from build123d import *

# Parameters (mm, degrees)
F1_DEPTH = 63.5
F2_DEPTH = 25.4
F3_DEPTH = 7.9375
F5_R     = 6.35


with BuildPart() as f1:
    # F0 (on Front) → F1 (new body, symmetric)
    with BuildSketch(Plane.XZ):
        Polygon((-41.275, -9.525), (41.275, -9.525), (41.275, 9.525), (22.225, 9.525), (-41.275, 9.525), align=None)
    extrude(amount=F1_DEPTH, both=True)

    # F0 (on Front) → F2 (join, symmetric)
    with BuildSketch(Plane.XZ):
        with BuildLine():
            Line((22.225, 9.525), (41.275, 9.525))
            Line((41.275, 9.525), (41.275, 27.0002))
            ThreePointArc((41.275, 27.0002), (45.9246798487, 38.2255201513), (57.15, 42.8752))
            Line((57.15, 42.8752), (60.325, 42.8752))
            Line((60.325, 42.8752), (60.325, 61.9252))
            Line((60.325, 61.9252), (57.15, 61.9252))
            add(Edge.make_bspline(
                [(53.8183914721, 61.765930391), (54.9540123477, 61.8314994044), (56.0654467047, 61.8844891287), (57.15, 61.9252)],
                knots=[108.0492715446, 108.0492715446, 108.0492715446, 108.0492715446, 111.5045361635, 111.5045361635, 111.5045361635, 111.5045361635], degree=3))
            ThreePointArc((53.8183914721, 61.765930391), (31.3032201925, 50.4884864122), (22.225, 27.0002))
            Line((22.225, 27.0002), (22.225, 9.525))
        make_face()
        Polygon((60.325, 61.9252), (60.325, 42.8752), (60.325, 38.1), (85.725, 38.1), (85.5438719422, 66.675), (60.325, 66.675), align=None)
    extrude(amount=F2_DEPTH, both=True)

    # F0 (on Front) → F3 (join, symmetric)
    with BuildSketch(Plane.XZ):
        with BuildLine():
            add(Edge.make_bspline(
                [(-41.275, 9.525), (-40.856674268, 45.3642172034), (18.3064924153, 59.7155276242), (53.8183914721, 61.765930391)],
                knots=[0, 0, 0, 0, 108.0492715446, 108.0492715446, 108.0492715446, 108.0492715446], degree=3))
            Line((-41.275, 9.525), (22.225, 9.525))
            Line((22.225, 9.525), (22.225, 27.0002))
            ThreePointArc((22.225, 27.0002), (31.3032201925, 50.4884864122), (53.8183914721, 61.765930391))
        make_face()
    extrude(amount=F3_DEPTH, both=True)

    # F0 (on Front) → F4 (revolve)
    with BuildSketch(Plane.XZ):
        Polygon((85.5438719422, 66.675), (85.725, 38.1), (111.125, 38.1), (111.125, 66.675), align=None)
    revolve(axis=Axis((85.6344359711, 0, 52.3875), (-0.0063385623, 0, 0.9999799111)))

    # F5
    f5_edges = [f1.edges().sort_by_distance(p)[0] for p in [
        (41.275, -63.5, 0),
        (-41.275, -63.5, 0),
        (-41.275, 63.5, 0),
        (41.275, 63.5, 0),
    ]]
    fillet(f5_edges, radius=F5_R)


solid = f1.part
Input: part model. Units: mm. Frame: model coordinates. A direction names the side the tool comes from. Coordinates: 2 decimals unless noted, no trailing zeros. Loops run counter-clockwise (first coordinate to the right, second up) from the corner with the lowest first, then second, coordinate; pieces in that order, holes last. Notation, with made-up numbers: (88, -9) -> (102, -9) arc R21 cw to (102, 27) -> close; hole circle Ø6 at (-8, -35). An arc over 180 degrees is marked (long way). Write item = value, one per line. Start each with the question number.
Item 1: Cut plane B-B, the plane y = -31. Return loops of the section in (x, z) (3 decimals).
Item 2: First-contact query: P1, Ø2.5, axis at x = 59, y = 5, coming from the +Z side; P2, Ø8, axis at x = 45.5, z = 44.5, coming from the +Y side; P3, Ø6, axis at x = 95, z = 54, coming from the -Y side. Flat tips, straight axial feed; report the tip coordinate or a pass-through.
Item 3: Cut plane A-A, the plane z = 0. Return loops of the section in (x, y) (3 decimals), plus the area to 3 significant figures.
Item 4: Reachability of faces 5 (the face through (45.8, -0.4, 38.1)), 6 (the face through (66, -19, 38.1)), 7 (the face through (22.225, -17, 18)), 8 (the face through (31.547, 16.547, 50.754)), 9 (the face through (87.2, 0.5, 38.1)) from +Z, -Z, +X, -X, +Y, -Y: full face, straight path, thin tool, end or side. Return the list, or none.
Item 5: Mould query, pull axis X, two halves, no side actions, for faces 1 (the face through (39.365, 61.689, 0.133)), 2 (the face through (60.325, 13, 41)), 3 (the face through (60.325, -6, 64)), 4 (the face through (73, 0, 66.675)). Classes: pulls with the +X half, pulls with the -X half, needs draft (parallel to the pull), parting line crosses it, or undercut.
Item 6: Material intervals for line 1 (Z direction, x = 19.5, y = -48) (3 decimals); line 2 (Y direction, x = 3.5, z = 40); line 3 (Y direction, x = 39, z = 26.5), sorted ascending.
Ans:
q1.outline = (-41.275, -9.525) -> (41.275, -9.525) -> (41.275, 9.525) -> (-41.275, 9.525) -> close
q2.P1 = 61.93
q2.P2 = 25.4
q2.P3 = -24.69
q3.outline = (-41.275, -57.15) arc R6.35 ccw to (-34.925, -63.5) -> (34.925, -63.5) arc R6.35 ccw to (41.275, -57.15) -> (41.275, 57.15) arc R6.35 ccw to (34.925, 63.5) -> (-34.925, 63.5) arc R6.35 ccw to (-41.275, 57.15) -> close
q3.area = 10,400 mm²
q4.face_5 = -Z, +Y, -Y
q4.face_6 = -Z, -Y
q4.face_7 = +Z, -X, -Y
q4.face_8 = +Z, -X, +Y
q4.face_9 = -Z, +X
q5.face_1 = pulls with the +X half
q5.face_2 = undercut
q5.face_3 = pulls with the -X half
q5.face_4 = needs draft
q6.line_1 = -9.525 to 9.525
q6.line_2 = -7.94 to 7.94
q6.line_3 = -25.4 to 25.4
